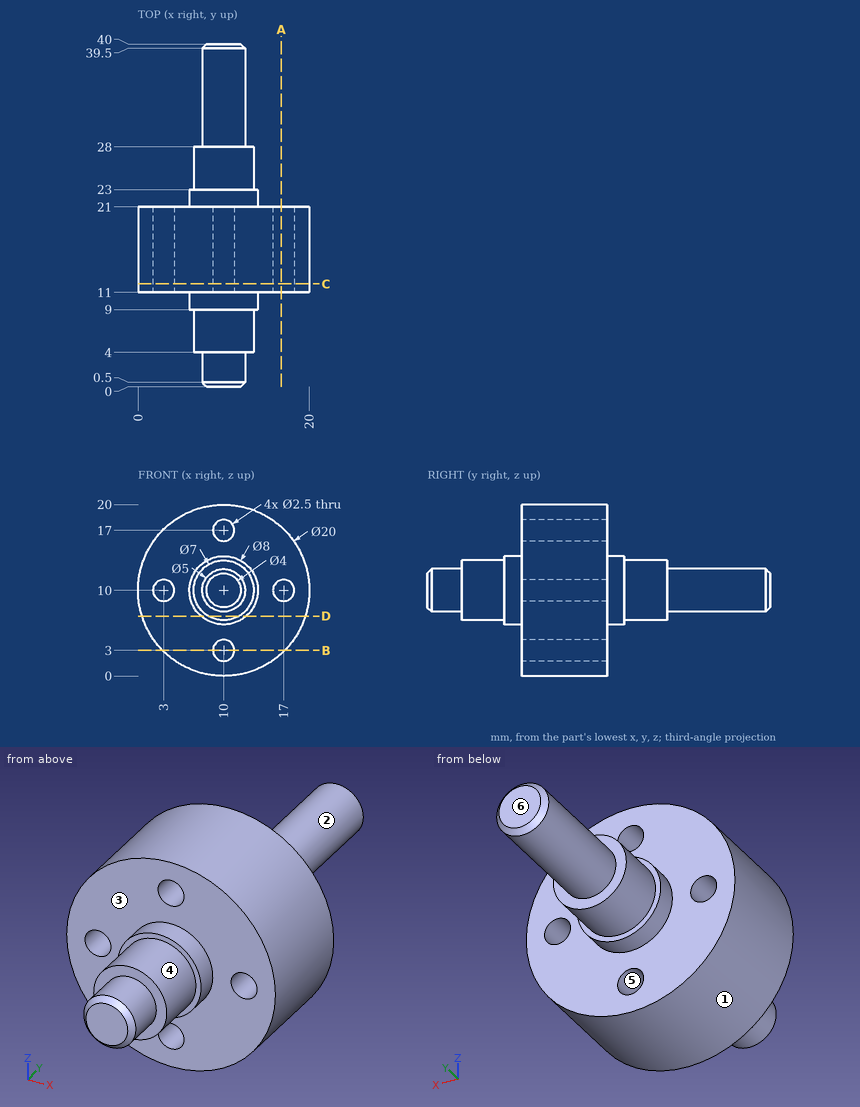
Can you work these out from the drawing? Everything is in mm from the part's minimum corner. A direction names the side the tool comes from. Give positions to 0.01 mm unless a question says otherwise; leave off trailing zeros. Order: outer loops, then holes, each group sorted by start corner. A loop starts at its lowest first (then second) coordinate and runs counter-clockwise, first axis right, second up.
Item 1: If we section it at B-B, the plane z = 3: Write out the boundary of the cut face in (x, y), plus the area to 3 significant figures.
Item 2: If we section it at D-D, the plane z = 7: Write out the boundary of the cut face in (x, y).
Item 3: I need wall thicknesses on line 1 (X direction, y = 14.75, z = 10); line 2 (Z direction, x = 10.25, y = 15.5); line 3 (X direction, y = 13.5, z = 17). Which ranges of each line are inside material? Lowest first, please.
Item 4: If we section it at A-A, the plane x = 16.75: Write out the boundary of the cut face in (y, z), plus the area to 3 significant figures.
Item 5: For the marked faces 1, 2 and 3, which set-ups out of +Z, -Z, +X, -X, +Y, -Y let a thin tool reach every point of the face, with its end or its side?
Item 6: If we section it at C-C, the plane y = 12: Write out the boundary of the cut face in (x, z), plus the area to 3 significant figures.
Item 7: I'm going to push flat-ended pins straight in: pin 1 (3 mm diameter, centred on x = 17, z = 14, fed in from +Y); pin 2 (4 mm diameter, centred on x = 5.5, y = 26.5, fed in from +Z); pin 3 (1.5 mm diameter, centred on x = 14.5, z = 10, fed in from -Y); pin 4 (2 mm diameter, centred on x = 10, z = 17, fed in from -Y). Where does each tip first touch, or does it pass through?
Item 8: If we mould it in two halves opening along Z, with no side actions, what happens to the marked faces 4, 5 and 6? For each: pulls with the +Z half, pulls with the -Z half, needs draft (parallel to the pull), parting line crosses it, or undercut.
Values:
1. outline: (2.86, 11) - (8.75, 11) - (8.75, 21) - (2.86, 21) - close; (11.25, 11) - (17.14, 11) - (17.14, 21) - (11.25, 21) - close
1. area: 118 mm2
2. outline: (0.46, 11) - (7.35, 11) - (7.35, 9) - (8.2, 9) - (8.2, 4) - (11.8, 4) - (11.8, 9) - (12.65, 9) - (12.65, 11) - (19.54, 11) - (19.54, 21) - (12.65, 21) - (12.65, 23) - (11.8, 23) - (11.8, 28) - (8.2, 28) - (8.2, 23) - (7.35, 23) - (7.35, 21) - (0.46, 21) - close
3. line 1: x = 0 to 1.75, 4.25 to 15.75, 18.25 to 20
3. line 2: z = 0 to 1.78, 4.22 to 15.78, 18.22 to 20
3. line 3: x = 2.86 to 8.75, 11.25 to 17.14
4. outline: (11, 2.62) - (21, 2.62) - (21, 8.78) - (11, 8.78) - close; (11, 11.22) - (21, 11.22) - (21, 17.38) - (11, 17.38) - close
4. area: 123 mm2
5. face 1: +Y, -Y
5. face 2: +Y
5. face 3: -Y
6. outline: circle Ø20 at (10, 10); hole circle Ø2.5 at (3, 10); hole circle Ø2.5 at (10, 3); hole circle Ø2.5 at (10, 17); hole circle Ø2.5 at (17, 10)
6. area: 295 mm2
7. pin 1: stops at y = 21
7. pin 2: stops at z = 12.45
7. pin 3: stops at y = 9
7. pin 4: passes through
8. face 4: parting line crosses it
8. face 5: undercut
8. face 6: needs draft
